Source: CAD feature listing. Evaluate the final solid. Frame: model axes, mm. A direction names the side the tool comes from. Round coordinates to 2 decimals unless told otherwise and drop trailing zeros. Write each loop counter-clockwise with the first axis right and the second up, starting at its lowest first coordinate (ties: lowest second). Pieces come first, ordered by that corner, then holes. Notation, with made-up numbers: M -26.75,-4.75 L -8.75,-4.75 A13 ccw -8.75,1.25 Z; hole C -17.5,34.5 d5. An arc over 180 degrees is marked long. Put each result on its own line as item: value. Start each with the question number.
```python
from build123d import *

# Parameters (mm, degrees)
SKETCH1_W           = 8
SKETCH1_H           = 17
SKETCH1_W_2         = 24
SKETCH1_H_2         = 8
BOSS_EXTRUDE1_DEPTH = 2
SKETCH4_W           = 3
SKETCH4_H           = 10
BOSS_EXTRUDE4_DEPTH = 36
BOSS_EXTRUDE5_REACH = 36.5
CUT_EXTRUDE3_DEPTH  = 38.5
SKETCH7_R           = 1.25
SKETCH7_R_2         = 1.5
CUT_EXTRUDE4_DEPTH  = 5


with BuildPart() as part:
    # Sketch1 → Boss-Extrude1 (new body)
    with BuildSketch(Plane(origin=(0, 0, 0), x_dir=(1, 0, 0), z_dir=(0, 1, 0))):
        with Locations((-17.713965849, 5.014073333)):
            Rectangle(SKETCH1_W, SKETCH1_H)
        with Locations((-1.713965849, 9.514073333)):
            Rectangle(SKETCH1_W_2, SKETCH1_H_2)
        with Locations((14.286034151, 5.014073333)):
            Rectangle(SKETCH1_W, SKETCH1_H)
    extrude(amount=-BOSS_EXTRUDE1_DEPTH)

    # Sketch4 → Boss-Extrude4 (add)
    with BuildSketch(Plane(origin=(0, -2, 0), x_dir=(-1, 0, 0), z_dir=(0, -1, 0))):
        with Locations((-14.286034151, 8.514073333)):
            Rectangle(SKETCH4_W, SKETCH4_H)
        with Locations((17.713965849, 8.514073333)):
            Rectangle(SKETCH4_W, SKETCH4_H)
    extrude(amount=BOSS_EXTRUDE4_DEPTH)

    # Sketch5 → Boss-Extrude5 (add, up to next)
    with BuildSketch(Plane.ZY.offset(-12.786034151), mode=Mode.PRIVATE) as boss_extrude5_sk1:
        Polygon((-13.514073333, -38), (-3.514073333, -32.226497308), (-3.514073333, -38), align=None)
    boss_extrude5_tool1 = extrude(boss_extrude5_sk1.sketch, amount=BOSS_EXTRUDE5_REACH, mode=Mode.PRIVATE) - part.part
    add(boss_extrude5_tool1.solids().sort_by_distance((12.786034, -36.075499, -6.847407))[0])

    # Sketch6 → Cut-Extrude3 (cut, through all)
    with BuildSketch(Plane.ZY.offset(19.213965849)):
        Polygon((-3.514073333, -38), (-3.514073333, -35), (-8.710225756, -38), align=None)
    extrude(amount=-CUT_EXTRUDE3_DEPTH, mode=Mode.SUBTRACT)

    # Sketch7 → Cut-Extrude4 (cut)
    with BuildSketch(Plane(origin=(0, 0, 0), x_dir=(1, 0, 0), z_dir=(0, 1, 0))):
        with Locations((-16.713965849, 9.014073333)):
            Circle(SKETCH7_R)
        with Locations((13.286034151, 9.014073333)):
            Circle(SKETCH7_R)
        with Locations((-17.963965849, -0.985926667)):
            Circle(SKETCH7_R_2)
        with Locations((14.536034151, -0.985926667)):
            Circle(SKETCH7_R_2)
    extrude(amount=-CUT_EXTRUDE4_DEPTH, mode=Mode.SUBTRACT)


solid = part.part
```
(1) Pull-direction query (X, two-part tool) for faces 1 (the flat face through (-2, -1, -5.514)), 2 (the flat face through (18.286, -1, -5)), 3 (the flat face through (-2, -2, -7)), 4 (the flat face through (-21.714, -1, -5)); classes: +X half, -X half, draft (parallel to the pull), parting line (faces both ways), or undercut.
(2) Ray query, line 1 along X through (y, z) = (-22.5, -6); line 2 along Y through (x, z) = (17, -0.75); line 3 along Z through (x, y) = (-16.5, -18.5). Return the intervals inside material, ascending.
(3) Section query A-A (x = 2). Return loops of the section in (y, z).
(4) Access query for faces 5 (the cylindrical face through (14.441, -2.465, -8.535)), 6 (the flat face through (-1.51, -35.15, -8.58)), 7 (the flat face through (-19.214, -20, -8)), 8 (the flat face through (10.286, -1, -1)). Directions: +Z, -Z, +X, -X, +Y, -Y. A direction counts if a zero-diameter tool reaches every point of the face in a straight line with its end or side. Return the directions, or none.
(5) Section query D-D (z = -7). Return loops of the section in (x, y).
(6) Contact query for flat-ended pins moving along their axis: P1, Ø3, axis at y = -18.5, z = -7, coming from the -X side; P2, Ø2.5, axis at x = -17.96, z = 0.99, coming from the -Y side; P3, Ø0.9, axis at x = -17, z = -8.5, coming from the +Y side; P4, Ø1, axis at x = -4, y = -1.5, coming from the +Z side. Output: stop coordinate, or through.
(7) Section query C-C (z = -9.5). Return loops of the section in (x, y).
(8) Section query B-B (y = -6). Return loops of the section in (x, z).
Entries:
1. face 1: undercut
1. face 2: +X half
1. face 3: undercut
1. face 4: -X half
2. line 1: -19.21 to -16.21, 12.79 to 15.79
2. line 2: -2 to 0
2. line 3: -13.51 to -3.51
3. outline: M -38,-13.51 L -32.23,-3.51 L -35,-3.51 L -38,-8.71 Z; M -2,-13.51 L 0,-13.51 L 0,-5.51 L -2,-5.51 Z
4. face 5: +Y
4. face 6: -Z
4. face 7: +Z, -Z, -X, -Y
4. face 8: +Z, +Y
5. outline: M -21.71,-2 L -19.21,-2 L -19.21,-37.01 L 15.79,-37.01 L 15.79,-2 L 18.29,-2 L 18.29,0 L -21.71,0 Z; hole M -16.21,-34.24 L 12.79,-34.24 L 12.79,-2 L -16.21,-2 Z
6. P1: x = -19.21
6. P2: through
6. P3: y = -5
6. P4: z = -5.51
7. outline: M -21.71,-2 L -19.21,-2 L -19.21,-38 L 15.79,-38 L 15.79,-2 L 18.29,-2 L 18.29,0 L 14.44,0 L 14.44,-5 L 12.79,-5 L 12.79,-35.68 L -16.21,-35.68 L -16.21,-5 L -17.87,-5 L -17.87,0 L -21.71,0 Z; M -15.56,-2 L 12.13,-2 L 12.13,0 L -15.56,0 Z
8. outline: M -19.21,-13.51 L -16.21,-13.51 L -16.21,-3.51 L -19.21,-3.51 Z; M 12.79,-13.51 L 15.79,-13.51 L 15.79,-3.51 L 12.79,-3.51 Z
